Autodesk Inventor part; units mm, degrees
ref_plane "YZ Plane" through (0, 0, 0) normal (1, 0, 0) x (0, 1, 0)
ref_plane "XZ Plane" through (0, 0, 0) normal (0, 1, 0) x (-1, 0, 0)
ref_plane "XY Plane" through (0, 0, 0) normal (0, 0, 1) x (1, 0, 0)
sketch "Sketch1" plane through (0, 0, 0) normal (0, 0, 1) x (1, 0, 0)
  line L0 (-14, -16) -> (14, -16)
  line L1 (14, -16) -> (14, -40)
  line L2 (14, -40) -> (24, -40)
  line L3 (24, -40) -> (24, -10)
  line L4 (24, -10) -> (9.2068, 7.6964)
  line L5 (-14, -16) -> (-14, -40)
  line L6 (-14, -40) -> (-24, -40)
  line L7 (-24, -40) -> (-24, -10)
  line L8 (-24, -10) -> (-9.2068, 7.6964)
  arc A0 (9.2068, 7.6964) -> (-9.2068, 7.6964) centre (0, 0) ccw
  circle A1 centre (0, 0) radius 7.5
  point P0 (0, -16)
  dimension "d0" = 28
  dimension "d1" = 10
  dimension "d2" = 24
  dimension "d3" = 40
  dimension "d4" = 30
  dimension "d5" = 15
  dimension "d6" = 12
extrude "Extrusion1" add sketch "Sketch1" along normal blind 12
sketch "Sketch2" plane through (24, -40, 0) normal (1, 0, 0) x (0, 0, -1)
  line L0 (0, 0) -> (0, 30) construction
  line L1 (0, 30) -> (-12, 30) construction
  line L2 (-12, 0) -> (-12, 30) construction
  line L3 (0, 0) -> (-12, 0) construction
  line L4 (0, 0) -> (-12, 0) construction
  line L5 (-6, 0) -> (-6, 10) construction
  circle A0 centre (-6, 10) radius 2.75
  point P0 (0, 40)
  dimension "d9" = 10
  dimension "d10" = 5.5
extrude "Extrusion2" cut sketch "Sketch2" against normal through all
sketch "Sketch3" plane through (0, 0, 12) normal (0, 0, 1) x (1, 0, 0)
  circle A0 centre (0, 0) radius 7.5
  arc A1 (9.2068, 7.6964) -> (-9.2068, 7.6964) centre (0, 0) ccw construction
  circle A2 centre (0, 0) radius 12
extrude "Extrusion3" add sketch "Sketch3" along normal blind 12
properties part number "con rod guide"
Work out the finished part from the listing and answer in its coordinate system (mm). A direction names the side the tool comes from. Coordinates: 2 decimals unless noted, no trailing zeros. Write each loop counter-clockwise with the first axis right and the second up, starting at its lowest first coordinate (ties: lowest second). Pieces come first, ordered by that corner, then holes.
Q1. Determine the mould class of faces 4 (the face through (-0.3, -15.8, 12)), 5 (the face through (-19, -40, 6)), 6 (the face through (-18.93, -27.273, 6.358)) for opening direction Y: released by +Y, released by -Y, zero draft, split by the parting line, or undercut.
Q2. A cutting plane is placed at B-B, the plane z = 2. Give the vertices of the cut face in (x, y), then the cut area to 3 significant figures.
Q3. Which of the six approach directions +Z, -Z, +X, -X, +Y, -Y give full straight-line access (tool end or side, diameter ignored) to faces 1 (the face through (-11.99, -0.53, 17.92)), 2 (the face through (0, -16, 6)), 3 (the face through (24, -25, 6))?
Q4. Find the intervals of material crossed by line 1 (X direction, y = -22, z = 4.5); line 2 (Y direction, x = 0, z = 13.75); line 3 (Z direction, x = 13, y = -8.5), in increasing order.
Q5. A cutting plane is placed at C-C, the plane z = 7.5. Give the vertices of the cut face in (x, y), then the cut area to 3 significant figures.
Q6. Each of these flat-tipped pins is pushed along its axis until it touches: pin 1 Ø5 at (y, z) = (-2, 6.5) entering from +X; pin 2 Ø5 at (x, z) = (10.5, 17) entering from -Y; pin 3 Ø5 at (x, z) = (13, 21.5) entering from +Y. Where does it stop, or does it pass through?
Q7. A cutting plane is placed at A-A, the plane y = -34. Give the vertices of the cut face in (x, z), then the cut area to 3 significant figures.
Findings below:
1. face 4: zero draft
1. face 5: released by -Y
1. face 6: undercut
2. outline: (-24, -40) - (-14, -40) - (-14, -16) - (14, -16) - (14, -40) - (24, -40) - (24, -10) - (9.21, 7.7) arc R12 ccw to (-9.21, 7.7) - (-24, -10) - close; hole circle Ø15 at (0, 0)
2. area: 1,230 mm2
3. face 1: +Z
3. face 2: +Z, -Z, -Y
3. face 3: +Z, -Z, +X, +Y, -Y
4. line 1: x = -24 to -14, 14 to 24
4. line 2: y = -12 to -7.5, 7.5 to 12
4. line 3: z = 0 to 12
5. outline: (-24, -40) - (-14, -40) - (-14, -32.3) - (-24, -32.3) - close; (-24, -27.7) - (-14, -27.7) - (-14, -16) - (14, -16) - (14, -27.7) - (24, -27.7) - (24, -10) - (9.21, 7.7) arc R12 ccw to (-9.21, 7.7) - (-24, -10) - close; (14, -40) - (24, -40) - (24, -32.3) - (14, -32.3) - close; hole circle Ø15 at (0, 0)
5. area: 1,140 mm2
6. pin 1: stops at x = 19.4
6. pin 2: stops at y = -8.94
6. pin 3: stops at y = 5.81
7. outline: (-24, 0) - (-14, 0) - (-14, 12) - (-24, 12) - close; (14, 0) - (24, 0) - (24, 12) - (14, 12) - close
7. area: 240 mm2
